Geometry check sheet. Reference: the model listing, model coordinates, mm. A direction names the side the tool comes from. Coordinates: 2 decimals unless noted, no trailing zeros. Write each loop counter-clockwise with the first axis right and the second up, starting at its lowest first coordinate (ties: lowest second). Pieces come first, ordered by that corner, then holes. Notation, with made-up numbers: M -16,63 L 24,63 A22 cw 24,70 Z; hole C -10,-36 d2. An arc over 180 degrees is marked long. Put each result on its own line as item: value. Start each with the question number.
1) Set-up check for faces 1 (the flat face through (-33, -43, 20)), 2 (the flat face through (-34.6, -43, 13)), 3 (the flat face through (-25, -65, 41)), 4 (the flat face through (-29, -21, 25)): record each of +Z, -Z, +X, -X, +Y, -Y from which the full face is reachable in a straight line by a thin tool's end or side.
2) Cross-section at C-C on z = 46.5. Record the cut outline in (x, y).
3) Cross-section at A-A on z = 17. Record the cut outline in (x, y), plus the area to 3 significant figures.
4) Scan lines: line 1 along X through (y, z) = (-7, 5.5); line 2 along X through (y, z) = (-12, 24); line 3 along Z through (x, y) = (-29.5, -23.5). Record each from-to range of solid material in increasing order.
5) Mould release check, pull along X, two halves, no side actions. Record for faces 5 (the flat face through (30.1, -43, 27)), 6 (the flat face through (0, -44, 7)), 7 (the flat face through (-37.996, -43, 17)): released by +X, released by -X, zero draft, split by the parting line, or undercut.
6) Cross-section at B-B on x = 6. Record the cut outline in (y, z).
7) Cross-section at D-D on z = 5.5. Record the cut outline in (x, y).
8) Gauge pin test, flat ends, axial feed: pin 1 (5 mm diameter, centred on x = -0.5, y = -75.5, fed in from +Z); pin 2 (1.3 mm diameter, centred on x = -24.5, z = 53, fed in from -Y); pin 3 (9 mm diameter, centred on x = -12, y = -28.5, fed in from +Z); pin 4 (6 mm diameter, centred on x = -6, z = 29.5, fed in from +Y). Record the tip position at first contact, or that the pin passes through.
from build123d import *

# Parameters (mm, degrees)
SKETCH_W        = 1.9
SKETCH_H        = 5
PAD_DEPTH       = 90
SKETCH001_W     = 2
SKETCH001_H     = 69
SKETCH001_H_2   = 73
POCKET_DEPTH    = 5
SKETCH002_W     = 60.2
SKETCH002_H     = 11.5
PAD001_DEPTH    = 2
SKETCH004_W     = 2
SKETCH004_H     = 2
PAD002_DEPTH    = 4
PAD003_DEPTH    = 92
SKETCH006_W     = 2
SKETCH006_H     = 73
PAD004_DEPTH    = 5
SKETCH007_W     = 2
SKETCH007_H     = 92
PAD005_DEPTH    = 38.74
SKETCH008_W     = 15
SKETCH008_H     = 75
POCKET001_DEPTH = 2
SKETCH009_W     = 2
SKETCH009_H     = 23
PAD006_DEPTH    = 38.74
SKETCH010_W     = 56.2
SKETCH010_H     = 2
PAD007_DEPTH    = 42.74
SKETCH011_W     = 56.2
SKETCH011_H     = 22
POCKET002_DEPTH = 2
SKETCH012_W     = 2
SKETCH012_H     = 15
PAD008_DEPTH    = 69
SKETCH013_W     = 2
SKETCH013_H     = 15
PAD009_DEPTH    = 90
PAD010_DEPTH    = 65


with BuildPart() as part:
    # Sketch → Pad (new body)
    with BuildSketch(Plane.XZ):
        Polygon((-30.1, 0), (30.1, 0), (30.1, 15.5), (28.1, 15.5), (28.1, 2), (-28.1, 2), (-28.1, 15.5), (-30.1, 15.5), align=None)
        with Locations((0, 4.5)):
            Rectangle(SKETCH_W, SKETCH_H)
        with Locations((-20.05, 4.5)):
            Rectangle(SKETCH_W, SKETCH_H)
        with Locations((20.05, 4.5)):
            Rectangle(SKETCH_W, SKETCH_H)
    extrude(amount=PAD_DEPTH)

    # Sketch001 (on Face3 of Pad) → Pocket (cut)
    with BuildSketch(Plane(origin=(0, 0, 15.5), x_dir=(-1, 0, 0), z_dir=(0, 0, 1))):
        with Locations((29.1, 55.5)):
            Rectangle(SKETCH001_W, SKETCH001_H)
        with Locations((-29.1, 53.5)):
            Rectangle(SKETCH001_W, SKETCH001_H_2)
    extrude(amount=-POCKET_DEPTH, mode=Mode.SUBTRACT)

    # Sketch002 (on Face2 of Pocket) → Pad001 (join)
    with BuildSketch(Plane(origin=(0, 0, 0), x_dir=(1, 0, 0), z_dir=(0, 1, 0))):
        with Locations((0, -5.75)):
            Rectangle(SKETCH002_W, SKETCH002_H)
    extrude(amount=PAD001_DEPTH)

    # Sketch004 → Pad002 (join)
    with BuildSketch(Plane(origin=(0, 0, 11.5), x_dir=(-1, 0, 0), z_dir=(0, 0, 1))):
        with Locations((-29.1, -1)):
            Rectangle(SKETCH004_W, SKETCH004_H)
        with Locations((29.1, -1)):
            Rectangle(SKETCH004_W, SKETCH004_H)
    extrude(amount=PAD002_DEPTH)

    # Sketch005 (on Face26 of Pad002) → Pad003 (join)
    with BuildSketch(Plane(origin=(0, 2, 0), x_dir=(1, 0, 0), z_dir=(0, 1, 0))):
        Polygon((-30.1, -54.24), (-30.1, 0), (-32.1, 0), (-32.1, -14.24), (-34.6, -14.24), (-34.6, -12.31), (-36.03, -12.31), (-37.995757, -14.275757), (-37.995757, -19.965757), (-36.03, -21.931514), (-34.6, -21.931514), (-34.6, -20), (-32.1, -20), (-32.1, -34.24), (-34.6, -34.24), (-34.6, -32.31), (-36.03, -32.31), (-37.995757, -34.275757), (-37.995757, -39.965757), (-36.03, -41.931514), (-34.6, -41.931514), (-34.6, -40.001514), (-32.1, -40.001514), (-32.1, -54.24), align=None)
    extrude(amount=-PAD003_DEPTH)

    # Sketch006 (on Face46 of Pad003) → Pad004 (join)
    with BuildSketch(Plane(origin=(0, 0, 10.5), x_dir=(-1, 0, 0), z_dir=(0, 0, 1))):
        with Locations((-29.1, 53.5)):
            Rectangle(SKETCH006_W, SKETCH006_H)
    extrude(amount=PAD004_DEPTH)

    # Sketch007 (on Face48 of Pad004) → Pad005 (join)
    with BuildSketch(Plane(origin=(0, 0, 15.5), x_dir=(-1, 0, 0), z_dir=(0, 0, 1))):
        with Locations((-29.1, 44)):
            Rectangle(SKETCH007_W, SKETCH007_H)
    extrude(amount=PAD005_DEPTH)

    # Sketch008 (on Face48 of Pad005) → Pocket001 (cut)
    with BuildSketch(Plane(origin=(30.1, 0, 0), x_dir=(0, 0, 1), z_dir=(1, 0, 0))):
        with Locations((18, 52.5)):
            Rectangle(SKETCH008_W, SKETCH008_H)
    extrude(amount=-POCKET001_DEPTH, mode=Mode.SUBTRACT)

    # Sketch009 (on Face51 of Pocket001) → Pad006 (join)
    with BuildSketch(Plane(origin=(0, 0, 15.5), x_dir=(-1, 0, 0), z_dir=(0, 0, 1))):
        with Locations((29.1, 9.5)):
            Rectangle(SKETCH009_W, SKETCH009_H)
    extrude(amount=PAD006_DEPTH)

    # Sketch010 (on Face17 of Pad006) → Pad007 (join)
    with BuildSketch(Plane(origin=(0, 0, 11.5), x_dir=(-1, 0, 0), z_dir=(0, 0, 1))):
        with Locations((0, -1)):
            Rectangle(SKETCH010_W, SKETCH010_H)
    extrude(amount=PAD007_DEPTH)

    # Sketch011 (on Face47 of Pad007) → Pocket002 (cut)
    with BuildSketch(Plane.XZ):
        with Locations((0, 22.5)):
            Rectangle(SKETCH011_W, SKETCH011_H)
    extrude(amount=-POCKET002_DEPTH, mode=Mode.SUBTRACT)

    # Sketch012 (on Face49 of Pocket002) → Pad008 (join)
    with BuildSketch(Plane.XZ.offset(21)):
        with Locations((-29.1, 46.74)):
            Rectangle(SKETCH012_W, SKETCH012_H)
    extrude(amount=PAD008_DEPTH)

    # Sketch013 (on Face26 of Pad008) → Pad009 (join)
    with BuildSketch(Plane.XZ):
        with Locations((27.1, 46.74)):
            Rectangle(SKETCH013_W, SKETCH013_H)
    extrude(amount=PAD009_DEPTH)

    # Sketch014 (on Face45 of Pad009) → Pad010 (join)
    with BuildSketch(Plane.XZ):
        Polygon((20.32, 39.24), (20.32, 43.44), (22.12, 43.44), (22.12, 41.24), (23.92, 41.24), (26.118204, 43.44), (26.118204, 39.24), align=None)
        Polygon((20.32, 54.24), (20.32, 50.04), (22.12, 50.04), (22.12, 52.24), (23.92, 52.24), (26.118204, 50.04), (26.118204, 54.24), align=None)
        Polygon((-22.32, 43.44), (-22.32, 39.24), (-28.12, 39.24), (-28.12, 43.438204), (-25.92, 41.24), (-24.12, 41.24), (-24.12, 43.44), align=None)
        Polygon((-22.32, 54.24), (-22.32, 50.04), (-24.12, 50.04), (-24.12, 52.24), (-25.92, 52.24), (-28.118204, 50.04), (-28.118204, 54.24), align=None)
    extrude(amount=PAD010_DEPTH)


solid = part.part
Answer key:
1. face 1: +Y, -Y
1. face 2: -Z, +Y, -Y
1. face 3: +Z, -Y
1. face 4: -Y
2. outline: M -32.1,-90 L -28.1,-90 L -28.1,0 L 26.1,0 L 26.1,-90 L 30.1,-90 L 30.1,2 L -32.1,2 Z
3. outline: M -38,-90 L -30.1,-90 L -30.1,-21 L -28.1,-21 L -28.1,2 L -38,2 Z; M 28.1,-15 L 30.1,-15 L 30.1,2 L 28.1,2 Z
3. area: 806 mm²
4. line 1: x = -32.1 to -28.1, -21 to -19.1, -0.95 to 0.95, 19.1 to 21, 28.1 to 30.1
4. line 2: x = -32.1 to -28.1, 28.1 to 30.1
4. line 3: z = 0 to 10.5, 39.24 to 54.24
5. face 5: released by +X
5. face 6: undercut
5. face 7: released by -X
6. outline: M -90,0 L 2,0 L 2,11.5 L 0,11.5 L 0,2 L -90,2 Z; M 0,33.5 L 2,33.5 L 2,54.24 L 0,54.24 Z
7. outline: M -32.1,-90 L -28.1,-90 L -28.1,0 L -21,0 L -21,-90 L -19.1,-90 L -19.1,0 L -0.95,0 L -0.95,-90 L 0.95,-90 L 0.95,0 L 19.1,0 L 19.1,-90 L 21,-90 L 21,0 L 28.1,0 L 28.1,-90 L 30.1,-90 L 30.1,2 L -32.1,2 Z
8. pin 1: stops at z = 7
8. pin 2: stops at y = -65
8. pin 3: stops at z = 2
8. pin 4: passes through
